Geometry check sheet. Reference: the model listing, model coordinates, mm. A direction names the side the tool comes from. Coordinates: 2 decimals unless noted, no trailing zeros. Write each loop counter-clockwise with the first axis right and the second up, starting at its lowest first coordinate (ties: lowest second). Pieces come first, ordered by that corner, then holes. Notation, with made-up numbers: (16, -32.5) -> (44, -32.5) arc R17 ccw to (44, -22.5) -> close; hole circle Ø4 at (31, -31.75). An arc over 180 degrees is marked (long way). Use a Markdown table: item, result.
```python
from build123d import *

# Parameters (mm, degrees)
F2_DEPTH = 5
F3_DEPTH = 5
F4_R     = 25.4
F4_R_2   = 16.4
F5_DEPTH = 5


with BuildPart() as f2:
    # F1 (on Top) → F2 (new body)
    with BuildSketch(Plane.XY):
        Polygon((34.5857864376, 54), (-34.5857864376, 54), (-54, 34.5857864376), (-54, -34.5857864376), (-34.5857864376, -54), (34.5857864376, -54), (54, -34.5857864376), (54, 34.5857864376), align=None)
        Polygon((46.5, 34.5857864376), (46.5, 3.75), (46.5, -3.75), (46.5, -34.5857864376), (34.5857864376, -46.5), (3.75, -46.5), (-3.75, -46.5), (-34.5857864376, -46.5), (-46.5, -34.5857864376), (-46.5, -3.75), (-46.5, 3.75), (-46.5, 34.5857864376), (-34.5857864376, 46.5), (-3.75, 46.5), (3.75, 46.5), (34.5857864376, 46.5), align=None, mode=Mode.SUBTRACT)
        with BuildLine():
            ThreePointArc((27.6468352619, -3.75), (27.8366368641, -1.8792679682), (27.9, 0))
            ThreePointArc((27.9, 0), (27.8366368641, 1.8792679682), (27.6468352619, 3.75))
            ThreePointArc((27.6468352619, 3.75), (19.7282791951, 19.7282791951), (3.75, 27.6468352619))
            ThreePointArc((3.75, 27.6468352619), (0, 27.9), (-3.75, 27.6468352619))
            ThreePointArc((-3.75, 27.6468352619), (-19.7282791951, 19.7282791951), (-27.6468352619, 3.75))
            ThreePointArc((-27.6468352619, 3.75), (-27.9, 0), (-27.6468352619, -3.75))
            ThreePointArc((-27.6468352619, -3.75), (-19.7282791951, -19.7282791951), (-3.75, -27.6468352619))
            ThreePointArc((-3.75, -27.6468352619), (0, -27.9), (3.75, -27.6468352619))
            ThreePointArc((3.75, -27.6468352619), (19.7282791951, -19.7282791951), (27.6468352619, -3.75))
        make_face()
        with BuildLine():
            ThreePointArc((7.4269778511, -19), (0, -20.4), (-7.4269778511, -19))
            ThreePointArc((-7.4269778511, -19), (-11.5032528408, 16.8474085272), (20.4, 0))
            ThreePointArc((20.4, 0), (16.8474085272, -11.5032528408), (7.4269778511, -19))
        make_face(mode=Mode.SUBTRACT)
        Polygon((-42.0710678119, 55), (-35, 55), (35, 55), (42.0710678119, 55), (37.0710678119, 60), (-37.0710678119, 60), align=None)
        Polygon((-55, 35), (-55, 42.0710678119), (-60, 37.0710678119), (-60, -37.0710678119), (-55, -42.0710678119), (-55, -35), align=None)
        Polygon((-42.0710678119, -55), (-37.0710678119, -60), (37.0710678119, -60), (42.0710678119, -55), (35, -55), (-35, -55), align=None)
        Polygon((60, 37.0710678119), (55, 42.0710678119), (55, 35), (55, -35), (55, -42.0710678119), (60, -37.0710678119), align=None)
        with BuildLine():
            ThreePointArc((27.6468352619, 3.75), (27.8366368641, 1.8792679682), (27.9, 0))
            ThreePointArc((27.9, 0), (27.8366368641, -1.8792679682), (27.6468352619, -3.75))
            Line((27.6468352619, -3.75), (46.5, -3.75))
            Line((46.5, -3.75), (46.5, 3.75))
            Line((46.5, 3.75), (27.6468352619, 3.75))
        make_face()
        with BuildLine():
            ThreePointArc((-3.75, 27.6468352619), (0, 27.9), (3.75, 27.6468352619))
            Line((3.75, 27.6468352619), (3.75, 46.5))
            Line((3.75, 46.5), (-3.75, 46.5))
            Line((-3.75, 46.5), (-3.75, 27.6468352619))
        make_face()
        with BuildLine():
            ThreePointArc((-27.6468352619, -3.75), (-27.9, 0), (-27.6468352619, 3.75))
            Line((-27.6468352619, 3.75), (-46.5, 3.75))
            Line((-46.5, 3.75), (-46.5, -3.75))
            Line((-46.5, -3.75), (-27.6468352619, -3.75))
        make_face()
        with BuildLine():
            Line((3.75, -46.5), (3.75, -27.6468352619))
            ThreePointArc((3.75, -27.6468352619), (0, -27.9), (-3.75, -27.6468352619))
            Line((-3.75, -27.6468352619), (-3.75, -46.5))
            Line((-3.75, -46.5), (3.75, -46.5))
        make_face()
        Polygon((-54, 36), (-36, 54), (-43.0710678119, 54), (-54, 43.0710678119), align=None)
        Polygon((-36, -54), (-54, -36), (-54, -43.0710678119), (-43.0710678119, -54), align=None)
        Polygon((54, -43.0710678119), (54, -36), (36, -54), (43.0710678119, -54), align=None)
        Polygon((43.0710678119, 54), (36, 54), (54, 36), (54, 43.0710678119), align=None)
        Polygon((-54, 34.5857864376), (-54, 36), (-55, 35), (-55, -35), (-54, -36), (-54, -34.5857864376), align=None)
        Polygon((34.5857864376, -54), (-34.5857864376, -54), (-36, -54), (-35, -55), (35, -55), (36, -54), align=None)
        Polygon((35, 55), (-35, 55), (-36, 54), (-34.5857864376, 54), (34.5857864376, 54), (36, 54), align=None)
        Polygon((55, 35), (54, 36), (54, 34.5857864376), (54, -34.5857864376), (54, -36), (55, -35), align=None)
        Polygon((-34.5857864376, -54), (-54, -34.5857864376), (-54, -36), (-36, -54), align=None)
        Polygon((-34.5857864376, 54), (-36, 54), (-54, 36), (-54, 34.5857864376), align=None)
        Polygon((54, -36), (54, -34.5857864376), (34.5857864376, -54), (36, -54), align=None)
        Polygon((54, 36), (36, 54), (34.5857864376, 54), (54, 34.5857864376), align=None)
        with BuildLine():
            ThreePointArc((3.9191835885, -19), (0, -19.4), (-3.9191835885, -19))
            Line((-3.9191835885, -19), (-7.4269778511, -19))
            ThreePointArc((-7.4269778511, -19), (0, -20.4), (7.4269778511, -19))
            Line((7.4269778511, -19), (3.9191835885, -19))
        make_face()
        Polygon((-36, 54), (-35, 55), (-42.0710678119, 55), (-43.0710678119, 54), align=None)
        Polygon((-55, 35), (-54, 36), (-54, 43.0710678119), (-55, 42.0710678119), align=None)
        Polygon((-54, -36), (-55, -35), (-55, -42.0710678119), (-54, -43.0710678119), align=None)
        Polygon((-35, -55), (-36, -54), (-43.0710678119, -54), (-42.0710678119, -55), align=None)
        Polygon((55, -42.0710678119), (55, -35), (54, -36), (54, -43.0710678119), align=None)
        Polygon((43.0710678119, -54), (36, -54), (35, -55), (42.0710678119, -55), align=None)
        Polygon((42.0710678119, 55), (35, 55), (36, 54), (43.0710678119, 54), align=None)
        Polygon((54, 43.0710678119), (54, 36), (55, 35), (55, 42.0710678119), align=None)
        with BuildLine():
            Line((3.9191835885, -19), (-3.9191835885, -19))
            ThreePointArc((-3.9191835885, -19), (0, -19.4), (3.9191835885, -19))
        make_face()
    extrude(amount=-F2_DEPTH)

    # F1 (on Top) → F3 (join)
    with BuildSketch(Plane.XY):
        Polygon((34.5857864376, 54), (-34.5857864376, 54), (-54, 34.5857864376), (-54, -34.5857864376), (-34.5857864376, -54), (34.5857864376, -54), (54, -34.5857864376), (54, 34.5857864376), align=None)
        Polygon((46.5, 34.5857864376), (46.5, 3.75), (46.5, -3.75), (46.5, -34.5857864376), (34.5857864376, -46.5), (3.75, -46.5), (-3.75, -46.5), (-34.5857864376, -46.5), (-46.5, -34.5857864376), (-46.5, -3.75), (-46.5, 3.75), (-46.5, 34.5857864376), (-34.5857864376, 46.5), (-3.75, 46.5), (3.75, 46.5), (34.5857864376, 46.5), align=None, mode=Mode.SUBTRACT)
        with BuildLine():
            ThreePointArc((27.6468352619, -3.75), (27.8366368641, -1.8792679682), (27.9, 0))
            ThreePointArc((27.9, 0), (27.8366368641, 1.8792679682), (27.6468352619, 3.75))
            ThreePointArc((27.6468352619, 3.75), (19.7282791951, 19.7282791951), (3.75, 27.6468352619))
            ThreePointArc((3.75, 27.6468352619), (0, 27.9), (-3.75, 27.6468352619))
            ThreePointArc((-3.75, 27.6468352619), (-19.7282791951, 19.7282791951), (-27.6468352619, 3.75))
            ThreePointArc((-27.6468352619, 3.75), (-27.9, 0), (-27.6468352619, -3.75))
            ThreePointArc((-27.6468352619, -3.75), (-19.7282791951, -19.7282791951), (-3.75, -27.6468352619))
            ThreePointArc((-3.75, -27.6468352619), (0, -27.9), (3.75, -27.6468352619))
            ThreePointArc((3.75, -27.6468352619), (19.7282791951, -19.7282791951), (27.6468352619, -3.75))
        make_face()
        with BuildLine():
            ThreePointArc((7.4269778511, -19), (0, -20.4), (-7.4269778511, -19))
            ThreePointArc((-7.4269778511, -19), (-11.5032528408, 16.8474085272), (20.4, 0))
            ThreePointArc((20.4, 0), (16.8474085272, -11.5032528408), (7.4269778511, -19))
        make_face(mode=Mode.SUBTRACT)
        with BuildLine():
            Line((3.75, -46.5), (3.75, -27.6468352619))
            ThreePointArc((3.75, -27.6468352619), (0, -27.9), (-3.75, -27.6468352619))
            Line((-3.75, -27.6468352619), (-3.75, -46.5))
            Line((-3.75, -46.5), (3.75, -46.5))
        make_face()
        with BuildLine():
            ThreePointArc((-27.6468352619, -3.75), (-27.9, 0), (-27.6468352619, 3.75))
            Line((-27.6468352619, 3.75), (-46.5, 3.75))
            Line((-46.5, 3.75), (-46.5, -3.75))
            Line((-46.5, -3.75), (-27.6468352619, -3.75))
        make_face()
        with BuildLine():
            ThreePointArc((27.6468352619, 3.75), (27.8366368641, 1.8792679682), (27.9, 0))
            ThreePointArc((27.9, 0), (27.8366368641, -1.8792679682), (27.6468352619, -3.75))
            Line((27.6468352619, -3.75), (46.5, -3.75))
            Line((46.5, -3.75), (46.5, 3.75))
            Line((46.5, 3.75), (27.6468352619, 3.75))
        make_face()
        with BuildLine():
            ThreePointArc((-3.75, 27.6468352619), (0, 27.9), (3.75, 27.6468352619))
            Line((3.75, 27.6468352619), (3.75, 46.5))
            Line((3.75, 46.5), (-3.75, 46.5))
            Line((-3.75, 46.5), (-3.75, 27.6468352619))
        make_face()
        with BuildLine():
            ThreePointArc((3.9191835885, -19), (0, -19.4), (-3.9191835885, -19))
            Line((-3.9191835885, -19), (-7.4269778511, -19))
            ThreePointArc((-7.4269778511, -19), (0, -20.4), (7.4269778511, -19))
            Line((7.4269778511, -19), (3.9191835885, -19))
        make_face()
        with BuildLine():
            Line((3.9191835885, -19), (-3.9191835885, -19))
            ThreePointArc((-3.9191835885, -19), (0, -19.4), (3.9191835885, -19))
        make_face()
    extrude(amount=F3_DEPTH)

    # F4 (on face) → F5 (join)
    with BuildSketch(Plane.XY.offset(5)):
        Circle(F4_R)
        with BuildLine():
            ThreePointArc((-7.4269778511, -19), (0, 20.4), (7.4269778511, -19))
            Line((7.4269778511, -19), (-7.4269778511, -19))
        make_face(mode=Mode.SUBTRACT)
        with BuildLine():
            Line((-7.4269778511, -19), (7.4269778511, -19))
            ThreePointArc((7.4269778511, -19), (0, 20.4), (-7.4269778511, -19))
        make_face()
        Circle(F4_R_2, mode=Mode.SUBTRACT)
    extrude(amount=F5_DEPTH)


solid = f2.part
```
Item 1: Section check C-C on y = 40.5. Record the boundary of the cut face in (x, z), then the cut area to 3 significant figures.
Answer block:
| item | result |
|---|---|
| outline | (-56.57, -5) -> (-40.59, -5) -> (-40.59, 5) -> (-48.09, 5) -> (-48.09, 0) -> (-56.57, 0) -> close; (-3.75, -5) -> (3.75, -5) -> (3.75, 5) -> (-3.75, 5) -> close; (40.59, -5) -> (56.57, -5) -> (56.57, 0) -> (48.09, 0) -> (48.09, 5) -> (40.59, 5) -> close |
| area | 310 mm^2 |
Item 2: Section check B-B on y = 0. Record the boundary of the cut face in (x, z).
Answer block:
| item | result |
|---|---|
| outline | (-60, -5) -> (-20.4, -5) -> (-20.4, 5) -> (-16.4, 5) -> (-16.4, 10) -> (-25.4, 10) -> (-25.4, 5) -> (-54, 5) -> (-54, 0) -> (-60, 0) -> close; (16.4, 5) -> (20.4, 5) -> (20.4, -5) -> (60, -5) -> (60, 0) -> (54, 0) -> (54, 5) -> (25.4, 5) -> (25.4, 10) -> (16.4, 10) -> close |
Item 3: Mould release check, pull along Y, two halves, no side actions. Record for faces 1 (the flat face through (54, 0, 2)), 2 (the flat face through (-44.429, -44.157, 2.465)), 3 (the flat face through (-46.5, 19, 0)): +Y half, -Y half, draft (parallel to the pull), parting line (faces both ways), or undercut.
Answer block:
| item | result |
|---|---|
| face 1 | draft |
| face 2 | -Y half |
| face 3 | undercut |
Item 4: Depth check by flat-ended pin: P1, Ø5.5, axis at y = 5.5, z = 2.5, coming from the -X side; P2, Ø1.5, axis at x = 28.5, z = 2.5, coming from the +Y side; P3, Ø10, axis at x = 6.5, y = -1.5, coming from the -Z side; P4, Ø1.5, axis at y = -5, z = 1.5, coming from the +X side. Enter the tip coordinate at first touch or a pass-through.
Answer block:
| item | result |
|---|---|
| P1 | stops at x = -60 |
| P2 | stops at y = 54 |
| P3 | passes through |
| P4 | stops at x = 54 |
Item 5: Tool access check on faces 4 (the flat face through (-48.375, 48.696, -2.465)), 5 (the flat face through (0, 54, 2)), 6 (the flat face through (-40.626, 40.459, -0.07)). Record the directions out of +Z, -Z, +X, -X, +Y, -Y that give a thin tool (end or side, any length) a straight path to the whole face; none if there is none.
Answer block:
| item | result |
|---|---|
| face 4 | +Z, -Z, -X, +Y |
| face 5 | +Z, +X, -X, +Y |
| face 6 | +Z, -Z |
Item 6: Section check A-A on x = 0. Record the boundary of the cut face in (y, z).
Answer block:
| item | result |
|---|---|
| outline | (-60, -5) -> (-19, -5) -> (-19, 5) -> (-16.4, 5) -> (-16.4, 10) -> (-25.4, 10) -> (-25.4, 5) -> (-54, 5) -> (-54, 0) -> (-60, 0) -> close; (16.4, 5) -> (20.4, 5) -> (20.4, -5) -> (60, -5) -> (60, 0) -> (54, 0) -> (54, 5) -> (25.4, 5) -> (25.4, 10) -> (16.4, 10) -> close |
Item 7: Section check D-D on x = 24. Record the boundary of the cut face in (y, z), then the cut area to 3 significant figures.
Answer block:
| item | result |
|---|---|
| outline | (-60, -5) -> (-46.5, -5) -> (-46.5, 5) -> (-54, 5) -> (-54, 0) -> (-60, 0) -> close; (-14.23, -5) -> (14.23, -5) -> (14.23, 5) -> (8.32, 5) -> (8.32, 10) -> (-8.32, 10) -> (-8.32, 5) -> (-14.23, 5) -> close; (46.5, -5) -> (60, -5) -> (60, 0) -> (54, 0) -> (54, 5) -> (46.5, 5) -> close |
| area | 578 mm^2 |
Item 8: Thickness scan on L1, parallel to Y at x = 32, z = 1.25; L2, parallel to Y at x = 0, z = 1.25; L3, parallel to Y at x = -8, z = 2.75. Record the ranges inside material, lowest first. Write a range as [from, to].
Answer block:
| item | result |
|---|---|
| L1 | y = [-54, -46.5], [-3.75, 3.75], [46.5, 54] |
| L2 | y = [-54, -19], [20.4, 54] |
| L3 | y = [-54, -46.5], [-26.73, -18.77], [18.77, 26.73], [46.5, 54] |
